Autodesk Inventor part; units mm, degrees
ref_plane "Arbeitsebene1" through (9.5, 0, 0) normal (1, 0, 0) x (0, 1, 0)
ref_plane "XZ Plane" through (0, 0, 0) normal (0, 1, 0) x (-1, 0, 0)
ref_plane "XY Plane" through (0, 0, 0) normal (0, 0, 1) x (1, 0, 0)
sketch "Skizze1" plane through (0, 0, 0) normal (0, 1, 0) x (-1, 0, 0)
  circle A0 centre (0, 0) radius 2.5
  dimension "d0" = 5
extrude "Extrusion1" add sketch "Skizze1" along normal blind 25
sketch "Skizze2" plane through (0, 25, 0) normal (0, 1, 0) x (1, 0, 0)
  circle A0 centre (0, 0) radius 2.5
  circle A1 centre (0, 0) radius 1.5
  dimension "d3" = 3
extrude "Extrusion2" cut sketch "Skizze2" against normal up to surface (25 mm away) contours A1
ref_plane "Arbeitsebene1" through (9.5, 0, 0) normal (1, 0, 0) x (0, 1, 0)
sketch "Skizze3" plane through (9.5, 0, 0) normal (1, 0, 0) x (0, 1, 0)
  circle A0 centre (12.5, 0) radius 2.5
  circle A1 centre (12.5, 0) radius 1.5
  point P0 (0, 0)
  dimension "d7" = 5
  dimension "d8" = 3
  dimension "d9" = 12.5
extrude "Extrusion3" add sketch "Skizze3" against normal up to surface
properties part number "divider" material "Messing, weicher Gelbton"
For this review, take the finished solid that the model builds, in its own axes (mm). A direction names the side the tool comes from. Give positions to 0.01 mm unless a question says otherwise; leave off trailing zeros. Loops run counter-clockwise (first coordinate to the right, second up) from the corner with the lowest first, then second, coordinate; pieces in that order, holes last. Notation, with made-up numbers: M 51.5,77.25 L 103.5,77.25 A25 ccw 103.5,90.25 Z; hole C 80,-9 d9. An arc over 180 degrees is marked long. One line per item, written item: value. Start each with the question number.
Q1. Machinability: for faces 1 (the face through (-1.5, 12.68, -0.07)), 2 (the face through (-2.31, 12.32, 0.96)), which of the approach directions +Z, -Z, +X, -X, +Y, -Y give a long, thin tool a straight path to every point of the face, cutting with its end or side? Answer none if there is none.
Q2. Draft analysis for pull direction Z (two halves, no side actions). For faces 3 (the face through (2.5, 12.5, 0)), 4 (the face through (5.802, 13.886, -0.575)), 5 (the face through (-2, 0, 0)), 6 (the face through (5.872, 14.885, 0.751)), state which applies: released by +Z, released by -Z, zero draft, split by the parting line, or undercut.
Q3. Add section A-A (z = 0). Give the boundary of the cut face in (x, y).
Q4. Add section C-C (x = 7.75). Give the boundary of the cut face in (y, z).
Q5. Add section D-D (z = -1.1). Give the boundary of the cut face in (x, y) (3 decimals).
Q6. Add section B-B (y = 12.5). Give the boundary of the cut face in (x, z), and give its area (3 significant figures).
Q7. For L1, parallel to Z at x = 5, y = 12.5; L2, parallel to Y at x = 5.75, z = 0, list the stretches that pass through material, from the lowest coordinate up.
Q8. Clearance check with flat-ended pins moving along their axes: pin 1 Ø2 at (x, y) = (-1.5, 13.5) entering from +Z; pin 2 Ø3 at (x, z) = (4, -1) entering from -Y; pin 3 Ø1 at (y, z) = (17.5, -2) entering from +X. State where each tip first meets the part, or that it passes through.
Reply:
1. face 1: +Y, -Y
1. face 2: none
2. face 3: undercut
2. face 4: undercut
2. face 5: zero draft
2. face 6: split by the parting line
3. outline: M -2.5,0 L -1.5,0 L -1.5,25 L -2.5,25 Z; M 1.5,0 L 2.5,0 L 2.5,10 L 9.5,10 L 9.5,11 L 2.5,11 L 2.5,14 L 9.5,14 L 9.5,15 L 2.5,15 L 2.5,25 L 1.5,25 Z
4. outline: C 12.5,0 d5; hole C 12.5,0 d3
5. outline: M -2.245,0 L -1.02,0 L -1.02,25 L -2.245,25 Z; M 1.02,0 L 2.245,0 L 2.245,10.255 L 9.5,10.255 L 9.5,11.48 L 2.245,11.48 L 2.245,13.52 L 9.5,13.52 L 9.5,14.745 L 2.245,14.745 L 2.245,25 L 1.02,25 Z
6. outline: M 0,-2.5 L 9.5,-2.5 L 9.5,-1.5 L 2,-1.5 A2.5 ccw 2,1.5 L 9.5,1.5 L 9.5,2.5 L 0,2.5 A2.5 ccw Z; hole C 0,0 d3
6. area: 28.8 mm²
7. L1: -2.5 to -1.5, 1.5 to 2.5
7. L2: 10 to 11, 14 to 15
8. pin 1: z = 2.45
8. pin 2: y = 10
8. pin 3: x = 2
